Work out the finished part from the listing and answer in its coordinate system (mm). Coordinates: 2 decimals unless noted, no trailing zeros. Order: outer loops, then holes, each group sorted by start corner. A loop starts at its lowest first (then second) coordinate and runs counter-clockwise, first axis right, second up. Notation, with made-up numbers: M -22,19.25 L -9,19.25 A33 cw -9,57.25 Z; hole C 25.25,22 d3. An arc over 180 degrees is marked long. Write item = value, one per line. Start each with the question number.
Q1. Find section B-B on z = 1659. Give the vertices of the cut face in (x, y), and give its area (3 significant figures).
Q2. Straight lines are drawn through the part: line 1 along Y through (x, z) = (52.25, 7.7); line 2 along Y through (x, z) = (52, 7); line 3 along X through (y, z) = (72.5, 279). For each, find the intervals that lie inside material, in ascending order.
Q3. Find section A-A on y = 58.5. Give the vertices of the cut face in (x, z).
Q4. Each of these flat-tipped pins is pushed along its axis until it touches: P1, Ø18.5, axis at y = 120, z = 494, coming from the +X side; P2, Ø5.5, axis at y = 24.45, z = -48, coming from the -X side; P3, Ø5, axis at y = 20, z = 1115.5, coming from the -X side. Where does it stop, or does it pass through?
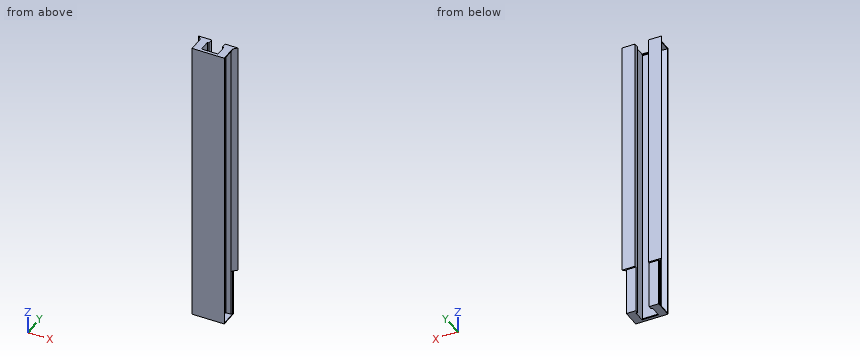
```python
from build123d import *

# Parameters (mm, degrees)
DODANIE_WYCI_GNI_CIE1_DEPTH = 1800
DODANIE_WYCI_GNI_CIE2_DEPTH = 348
DODANIE_WYCI_GNI_CIE3_DEPTH = 7
DODANIE_WYCI_GNI_CIE5_DEPTH = 7
ZAOKR_GLENIE1_R             = 5
SZKIC16_R                   = 3
WYTNIJ_WYCI_GNI_CIE1_DEPTH  = 10.2


with BuildPart() as part:
    # Szkic4 → Dodanie-wyciągnięcie1 (new body)
    with BuildSketch(Plane.XY):
        Polygon((0, 0), (0, 5), (48.5, 9), (48.5, 107), (6.5, 111), (-26.5, 144), (70.2, 144), (70.2, 107), (58.679571348, 107), (58.679571348, 13), (181.3, 13), (181.3, 107), (169.8, 107), (169.8, 144), (266.5, 144), (233.5, 111), (191.5, 107), (191.5, 9), (240, 5), (240, 0), align=None)
    extrude(amount=DODANIE_WYCI_GNI_CIE1_DEPTH)

    # Szkic5 → Dodanie-wyciągnięcie2 (add)
    with BuildSketch(Plane.XY):
        Polygon((0, 0), (0, 5), (48.5, 9), (48.5, 107), (6.5, 111), (0, 117.5), (0, 133), (6.5, 133), (70.2, 133), (70.2, 107), (58.679571348, 107), (58.679571348, 13), (181.3, 13), (181.3, 107), (169.8, 107), (169.8, 133), (233.5, 133), (240, 133), (240, 118.39460416), (233.5, 111), (191.5, 107), (191.5, 9), (240, 5), (240, 0), align=None)
    extrude(amount=-DODANIE_WYCI_GNI_CIE2_DEPTH)

    # Szkic10 → Dodanie-wyciągnięcie3 (add)
    with BuildSketch(Plane.XY.offset(-348)):
        Polygon((0, 0), (0, 117.5), (0, 133), (6.5, 133), (70.2, 133), (70.2, 107), (58.679571348, 107), (58.679571348, 22.5), (181.3, 22.5), (181.3, 107), (169.8, 107), (169.8, 133), (233.5, 133), (240, 133), (240, 118.39460416), (240, 0), align=None)
    extrude(amount=-DODANIE_WYCI_GNI_CIE3_DEPTH)

    # Szkic11 → Dodanie-wyciągnięcie5 (add)
    with BuildSketch(Plane.XY.offset(1800)):
        Polygon((0, 0), (0, 5), (0, 117.5), (-26.5, 144), (70.2, 144), (70.2, 107), (58.679571348, 107), (58.679571348, 22.5), (181.3, 22.5), (181.3, 107), (169.8, 107), (169.8, 144), (266.5, 144), (240, 117.5), (240, 5), (240, 0), align=None)
    extrude(amount=DODANIE_WYCI_GNI_CIE5_DEPTH)

    # Zaokrąglenie1
    zaokr_glenie1_edges = [part.edges().sort_by_distance(p)[0] for p in [
        (48.5, 107, 726),
        (48.5, 9, 726),
        (191.5, 9, 726),
        (191.5, 107, 726),
    ]]
    fillet(zaokr_glenie1_edges, radius=ZAOKR_GLENIE1_R)

    # Szkic16 → Wytnij-wyciągnięcie1 (cut)
    with BuildSketch(Plane.ZY.offset(-48.5)):
        with Locations((-48, 90.453565926)):
            Circle(SZKIC16_R)
        with Locations((7.7, 90.453565926)):
            Circle(SZKIC16_R)
        with Locations((7.7, 24.453565926)):
            Circle(SZKIC16_R)
        with Locations((-48, 24.453565926)):
            Circle(SZKIC16_R)
    extrude(amount=-WYTNIJ_WYCI_GNI_CIE1_DEPTH, mode=Mode.SUBTRACT)


solid = part.part
```
Findings below:
q1.outline = M -26.5,144 L 6.5,111 L 43.97,107.43 A5 cw 48.5,102.45 L 48.5,13.6 A5 cw 43.91,8.62 L 0,5 L 0,0 L 240,0 L 240,5 L 196.09,8.62 A5 cw 191.5,13.6 L 191.5,102.45 A5 cw 196.03,107.43 L 233.5,111 L 266.5,144 L 169.8,144 L 169.8,107 L 181.3,107 L 181.3,13 L 58.68,13 L 58.68,107 L 70.2,107 L 70.2,144 Z
q1.area = 10,100 mm^2
q2.line_1 = 0 to 21.45, 27.45 to 87.45, 93.45 to 144
q2.line_2 = 0 to 21.54, 27.37 to 87.54, 93.37 to 144
q2.line_3 = 48.5 to 58.68, 181.3 to 191.5
q3.outline = M 0,-355 L 58.68,-355 L 58.68,1807 L 0,1807 L 0,1800 L 48.5,1800 L 48.5,-348 L 0,-348 Z; M 181.3,-355 L 240,-355 L 240,-348 L 191.5,-348 L 191.5,1800 L 240,1800 L 240,1807 L 181.3,1807 Z
q4.P1 = 251.75
q4.P2 = 181.3
q4.P3 = 48.5
